The model under review builds one solid part; all positions refer to its coordinate system, in mm. A direction names the side the tool comes from. Coordinates: 2 decimals unless noted, no trailing zeros. Order: outer loops, then holes, each group sorted by start corner. A loop starts at its lowest first (then second) coordinate and runs counter-clockwise, first axis right, second up. Notation, with made-up numbers: M 60,-26 L 80,-26 A6 cw 80,-15 Z; hole C 22,-34.75 d6. An arc over 180 degrees is marked long. Write each question's results on one line, items separated by ' | '.
from build123d import *

# Parameters (mm, degrees)
F1_DEPTH = 50.8
F2_R     = 7.9375
F3_DEPTH = 38.101
F4_R     = 7.9375
F5_DEPTH = 12.7


with BuildPart() as f1:
    # F0 (on Front) → F1 (new body)
    with BuildSketch(Plane.XZ):
        Polygon((-31.75, -19.05), (31.75, -19.05), (31.75, -12.7), (25.4, -12.7), (25.4, 12.7), (31.75, 12.7), (31.75, 19.05), (-31.75, 19.05), (-31.75, 12.7), (-25.4, 12.7), (-25.4, -12.7), (-31.75, -12.7), align=None)
    extrude(amount=F1_DEPTH)

    # F2 (on face) → F3 (cut, through all)
    with BuildSketch(Plane.XY.offset(19.05)):
        with Locations((0, -25.4)):
            Circle(F2_R)
    extrude(amount=-F3_DEPTH, mode=Mode.SUBTRACT)

    # F4 (on face) → F5 (cut)
    with BuildSketch(Plane(origin=(0, 0, 0), x_dir=(-1, 0, 0), z_dir=(0, 1, 0))):
        Circle(F4_R)
    extrude(amount=-F5_DEPTH, mode=Mode.SUBTRACT)


solid = f1.part
1) Take a section at C-C on z = 0. State the section outline as (x, y) points (1 decimal).
Solutions:
outline: M -25.4,-50.8 L 25.4,-50.8 L 25.4,0 L 7.9,0 L 7.9,-12.7 L -7.9,-12.7 L -7.9,0 L -25.4,0 Z; hole C 0,-25.4 d15.9
2) For pin 1 (1.5 mm diameter, centred on y = -18, z = 4, fed in from -X); pin 2 (7.5 mm diameter, centred on y = -27, z = 3, fed in from +X); pin 3 (14.5 mm diameter, centred on x = 0, y = -25.4, fed in from +Z); pin 4 (12.5 mm diameter, centred on x = 0, z = 0, fed in from +Y), all flat-tipped, find the tip position at first contact; note any pin that passes through.
Solutions:
pin 1: x = -25.4 | pin 2: x = 25.4 | pin 3: through | pin 4: y = -12.7
3) To check wall thickness, follow line 1 along Z through (x, y) = (0, -7.75); line 2 along X through (y, z) = (-25, 11); line 3 along Y through (x, z) = (0, 7). State the ranges of each line that lie inside material, in increasing order.
Solutions:
line 1: -19.05 to -7.94, 7.94 to 19.05 | line 2: -25.4 to -7.93, 7.93 to 25.4 | line 3: -50.8 to -33.34, -17.46 to -12.7
4) For faces 4 (the flat face through (-31.75, -25, 16)), 5 (the flat face through (-29, -25, 12.7)), 6 (the flat face through (29, -25, -12.7)), 7 (the flat face through (0, -12.7, 0)), 8 (the flat face through (7, -31, -19.05)), list the 3-axis set-ups (+Z, -Z, +X, -X, +Y, -Y) from which the entire face can be reached by the end or side of a thin tool; tool diameter is ignored.
Solutions:
face 4: +Z, -Z, -X, +Y, -Y | face 5: -X, +Y, -Y | face 6: +X, +Y, -Y | face 7: +Y | face 8: -Z, +X, -X, +Y, -Y
5) Take a section at A-A on y = -25.4. State the section outline as (x, z) points, plus the area to 3 significant figures.
Solutions:
outline: M -31.75,-19.05 L -7.94,-19.05 L -7.94,19.05 L -31.75,19.05 L -31.75,12.7 L -25.4,12.7 L -25.4,-12.7 L -31.75,-12.7 Z; M 7.94,-19.05 L 31.75,-19.05 L 31.75,-12.7 L 25.4,-12.7 L 25.4,12.7 L 31.75,12.7 L 31.75,19.05 L 7.94,19.05 Z | area: 1,490 mm2
6) The part is to be moulded in two halves that separate along Z. For faces 1 (the flat face through (31.75, -25, -16)), 2 (the flat face through (-7, -31, 19.05)), 3 (the flat face through (29, -25, 12.7)), say which applies: pulls with the +Z half, pulls with the -Z half, needs draft (parallel to the pull), parting line crosses it, or undercut.
Solutions:
face 1: needs draft | face 2: pulls with the +Z half | face 3: undercut
7) Take a section at B-B on x = 27. State the section outline as (y, z) points, plus the area to 3 significant figures.
Solutions:
outline: M -50.8,-19.05 L 0,-19.05 L 0,-12.7 L -50.8,-12.7 Z; M -50.8,12.7 L 0,12.7 L 0,19.05 L -50.8,19.05 Z | area: 645 mm2
